Autodesk Inventor part; units mm, degrees
ref_plane "YZ Plane" through (0, 0, 0) normal (1, 0, 0) x (0, 1, 0)
ref_plane "XZ Plane" through (0, 0, 0) normal (0, 1, 0) x (-1, 0, 0)
ref_plane "XY Plane" through (0, 0, 0) normal (0, 0, 1) x (1, 0, 0)
sketch "Sketch1" plane through (0, 0, 0) normal (0, 0, 1) x (1, 0, 0)
  line L0 (0, 0) -> (-15, 0) construction
  line L1 (0, 0) -> (0, 3)
  line L2 (-15, 3) -> (0, 3) construction
  line L3 (-15, 0) -> (-15, 3) construction
  line L4 (15, 0) -> (15, 3)
  line L5 (15, 9) -> (-15, 9)
  line L6 (-15, -11) -> (15, -11)
  line L7 (15, -11) -> (15, 9)
  line L8 (0, 3) -> (15, 3)
  line L9 (0, 0) -> (15, 0)
  line L10 (0, 3) -> (0, 0)
  line L11 (15, 3) -> (15, 0)
  line L12 (-15, 9) -> (-32, 9)
  line L13 (-32, 9) -> (-32, -31)
  line L14 (-15, -11) -> (-24.3262, -31)
  line L15 (-15, -11) -> (7.0676, -11) construction
  line L16 (-24.3262, -31) -> (-32, -31)
  line L17 (-32, 1) -> (-38, 1)
  line L18 (-38, 1) -> (-38, -23)
  line L19 (-38, -23) -> (-32, -23)
  line L20 (-32, -23) -> (-32, 1)
  dimension "d0" = 20
  dimension "d1" = 6
  dimension "d3" = 15
  dimension "d4" = 17
  dimension "d5" = 40
  dimension "d6" = 115
  dimension "d7" = 47
  dimension "d8" = 6
  dimension "d9" = 8
  dimension "d10" = 8
extrude "Extrusion1" add sketch "Sketch1" along normal blind 3 contours L9 L7 L6 L14 L16 L13 L12 L5 L8 L1 | L13 L19 L18 L17
sketch "Sketch2" plane through (0, 0, 0) normal (0, 0, -1) x (-1, 0, 0)
  line L0 (26, -18.5) -> (29, -18.5)
  line L1 (29, -18.5) -> (29, -3.5)
  line L2 (29, -3.5) -> (26, -3.5)
  line L3 (26, -3.5) -> (26, -18.5)
  line L4 (-15, 9) -> (32, 9)
  line L5 (32, 9) -> (32, 1)
  point P0 (0, 0)
  dimension "d13" = 3
  dimension "d14" = 15
  dimension "d15" = 12.5
  dimension "d16" = 3
extrude "Extrusion2" cut sketch "Sketch2" against normal blind 3
properties part number "Camera bracket raiser"
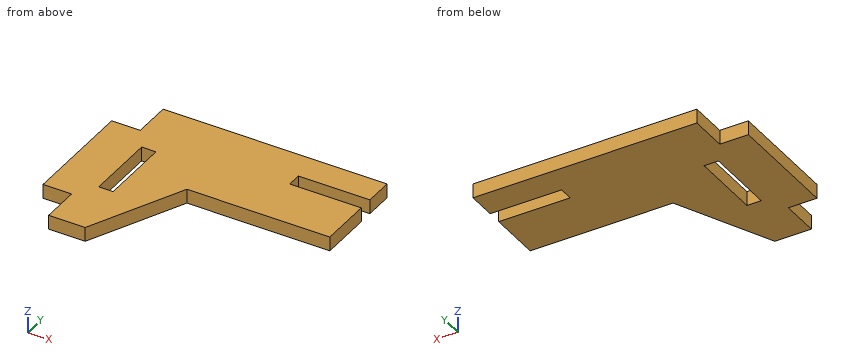
The listing builds one solid part. Answer for the finished solid, in the listing's coordinates (mm). Coordinates: 2 decimals unless noted, no trailing zeros. Order: outer loops, then holes, each group sorted by start corner. A loop starts at its lowest first (then second) coordinate and runs counter-clockwise, first axis right, second up. Notation, with made-up numbers: M 14.25,50 L 26.25,50 A34 cw 26.25,82 Z; hole C 59,22 d7. An arc over 180 degrees is marked long. Answer as a JSON object with one key per item and string values. Group by question number.
1. Section B-B on x = 5 is taken. Write down the section's boundary in (y, z).
2. Flat-ended cylindrical pins translate along their axes: P1, Ø10, axis at x = 0.5, y = -18, coming from the +Z side; P2, Ø1.5, axis at y = -26.5, z = 1, coming from the -X side; P3, Ø1.5, axis at y = 1.5, z = 1.5, coming from the +X side; P4, Ø1.5, axis at x = -36, z = 1, coming from the -Y side. Find the tip coordinate at first contact, or state that the pin passes through.
3. Section C-C on x = -35 is taken. Write down the section's boundary in (y, z), then the cut area to 3 significant figures.
4. Straight lines are drawn through the part: line 1 (Y direction, x = -28.5, z = 1); line 2 (Y direction, x = 10, z = 2.85); line 3 (Y direction, x = -0.5, z = 1). For each, find the intervals that lie inside material, in ascending order.
5. Section D-D on y = -25 is taken. Write down the section's boundary in (x, z), then the cut area to 3 significant figures.
6. Section A-A on z = 1.05 is taken. Write down the section's boundary in (x, y).
Values follow:
{
 "1": {"outline": "M -11,0 L 0,0 L 0,3 L -11,3 Z; M 3,0 L 9,0 L 9,3 L 3,3 Z"},
 "2": {"P1": "through", "P2": "x = -32", "P3": "x = 0", "P4": "y = -23"},
 "3": {"outline": "M -23,0 L 1,0 L 1,3 L -23,3 Z", "area": "72.0 mm2"},
 "4": {"line 1": "-31 to -18.5, -3.5 to 9", "line 2": "-11 to 0, 3 to 9", "line 3": "-11 to 9"},
 "5": {"outline": "M -32,0 L -21.53,0 L -21.53,3 L -32,3 Z", "area": "31.4 mm2"},
 "6": {"outline": "M -38,-23 L -32,-23 L -32,-31 L -24.33,-31 L -15,-11 L 15,-11 L 15,0 L 0,0 L 0,3 L 15,3 L 15,9 L -32,9 L -32,1 L -38,1 Z; hole M -29,-18.5 L -26,-18.5 L -26,-3.5 L -29,-3.5 Z"}
}
